Verification items for the finished model (mm, model axes). A direction names the side the tool comes from. Coordinates: 2 decimals unless noted, no trailing zeros. Write each loop counter-clockwise with the first axis right and the second up, starting at its lowest first coordinate (ties: lowest second). Pieces come first, ordered by that corner, then holes. Notation, with made-up numbers: (-36, -29.5) -> (-1, -29.5) arc R25 cw to (-1, 1.5) -> close; hole circle Ø7 at (10, 56). An arc over 180 degrees is marked (long way). Use a Markdown table: item, result. Add a question column.
from build123d import *

# Parameters (mm, degrees)
BOSS_EXTRUDE1_DEPTH = 2.7


with BuildPart() as part:
    # Sketch1 → Boss-Extrude1 (new body)
    with BuildSketch(Plane.XY):
        with BuildLine():
            Line((7.975, 17.5), (7.066267392, 17.5))
            ThreePointArc((7.066267392, 17.5), (5.52829673, 17.075780705), (4.425283954, 15.923097495))
            Line((4.425283954, 15.923097495), (-10.076639064, -10.98956215))
            ThreePointArc((-10.076639064, -10.98956215), (-10.52310248, -12.138320442), (-10.675, -13.361391307))
            Line((-10.675, -13.361391307), (-10.675, -14.8))
            Line((-10.675, -14.8), (-6.945, -14.8))
            Line((-6.945, -14.8), (-6.945, -17.5))
            Line((-6.945, -17.5), (-3.215, -17.5))
            Line((-3.215, -17.5), (-3.215, -14.8))
            Line((-3.215, -14.8), (0.515, -14.8))
            Line((0.515, -14.8), (0.515, -17.5))
            Line((0.515, -17.5), (4.245, -17.5))
            Line((4.245, -17.5), (4.245, -14.8))
            Line((4.245, -14.8), (7.975, -14.8))
            Line((7.975, -14.8), (7.975, -10.185714286))
            Line((7.975, -10.185714286), (10.675, -10.185714286))
            Line((10.675, -10.185714286), (10.675, -5.571428571))
            Line((10.675, -5.571428571), (7.975, -5.571428571))
            Line((7.975, -5.571428571), (7.975, -0.957142857))
            Line((7.975, -0.957142857), (10.675, -0.957142857))
            Line((10.675, -0.957142857), (10.675, 3.657142857))
            Line((10.675, 3.657142857), (7.975, 3.657142857))
            Line((7.975, 3.657142857), (7.975, 8.271428571))
            Line((7.975, 8.271428571), (10.675, 8.271428571))
            Line((10.675, 8.271428571), (10.675, 12.885714286))
            Line((10.675, 12.885714286), (7.975, 12.885714286))
            Line((7.975, 12.885714286), (7.975, 17.5))
        make_face()
    extrude(amount=-BOSS_EXTRUDE1_DEPTH)


solid = part.part
1) Cross-section at D-D on x = -1.75. Record the boundary of the cut face in (y, z).
2) Set-up check for faces 4 (the face through (7.975, 15, -1)), 5 (the face through (9, -0.957, -1)), 6 (the face through (9, -10.186, -1)), 7 (the face through (-6.945, -16, -1)): record each of +Z, -Z, +X, -X, +Y, -Y from which the full face is reachable in a straight line by a thin tool's end or side.
3) Cross-section at C-C on y = -2.5. Record the boundary of the cut face in (x, z) (3 decimals), then the cut area to 3 significant figures.
4) Cross-section at A-A on x = 8.75. Record the boundary of the cut face in (y, z), then the cut area to 3 significant figures.
5) Cross-section at B-B on z = -1.05. Record the boundary of the cut face in (x, y) (3 decimals), then the cut area to 3 significant figures.
6) Release check for a two-part mould opening along X. For faces 1 (the face through (4.245, -16, -1)), 2 (the face through (-3.215, -16, -1)), 3 (the face through (2, -4, -2.7)) record: released by +X, released by -X, zero draft, split by the parting line, or undercut.
7) Thickness scan on L1, parallel to Y at x = 9, z = -1.4; L2, parallel to Y at x = 7.25, z = -0.25; L3, parallel to Y at x = -7.75, z = -2.35. Record the ranges inside material, lowest first.
8) Gauge pin test, flat ends, axial feed: pin 1 (1.4 mm diameter, centred on x = 9.5, z = -1.5, fed in from +Y); pin 2 (1.3 mm diameter, centred on y = -16.5, z = -2, fed in from -X) (3 decimals); pin 3 (1.4 mm diameter, centred on x = -8.5, z = -1, fed in from -Y); pin 4 (5 mm diameter, centred on x = -6.5, y = 3.5, fed in from +Z). Record the tip position at first contact, or that the pin passes through.
Returned:
| question | item | result |
|---|---|---|
| 1 | outline | (-14.8, -2.7) -> (4.46, -2.7) -> (4.46, 0) -> (-14.8, 0) -> close |
| 2 | face 4 | +Z, -Z, +X, +Y |
| 2 | face 5 | +Z, -Z, +X |
| 2 | face 6 | +Z, -Z, +X, -Y |
| 2 | face 7 | +Z, -Z, -X, -Y |
| 3 | outline | (-5.502, -2.7) -> (7.975, -2.7) -> (7.975, 0) -> (-5.502, 0) -> close |
| 3 | area | 36.4 mm² |
| 4 | outline | (-10.19, -2.7) -> (-5.57, -2.7) -> (-5.57, 0) -> (-10.19, 0) -> close; (-0.96, -2.7) -> (3.66, -2.7) -> (3.66, 0) -> (-0.96, 0) -> close; (8.27, -2.7) -> (12.89, -2.7) -> (12.89, 0) -> (8.27, 0) -> close |
| 4 | area | 37.4 mm² |
| 5 | outline | (-10.675, -14.8) -> (-6.945, -14.8) -> (-6.945, -17.5) -> (-3.215, -17.5) -> (-3.215, -14.8) -> (0.515, -14.8) -> (0.515, -17.5) -> (4.245, -17.5) -> (4.245, -14.8) -> (7.975, -14.8) -> (7.975, -10.186) -> (10.675, -10.186) -> (10.675, -5.571) -> (7.975, -5.571) -> (7.975, -0.957) -> (10.675, -0.957) -> (10.675, 3.657) -> (7.975, 3.657) -> (7.975, 8.271) -> (10.675, 8.271) -> (10.675, 12.886) -> (7.975, 12.886) -> (7.975, 17.5) -> (7.066, 17.5) arc R3 ccw to (4.425, 15.923) -> (-10.077, -10.99) arc R5 ccw to (-10.675, -13.361) -> close |
| 5 | area | 423 mm² |
| 6 | face 1 | released by +X |
| 6 | face 2 | undercut |
| 6 | face 3 | zero draft |
| 7 | L1 | y = -10.19 to -5.57, -0.96 to 3.66, 8.27 to 12.89 |
| 7 | L2 | y = -14.8 to 17.5 |
| 7 | L3 | y = -14.8 to -6.67 |
| 8 | pin 1 | stops at y = 12.89 |
| 8 | pin 2 | stops at x = -6.945 |
| 8 | pin 3 | stops at y = -14.8 |
| 8 | pin 4 | passes through |
